Part model, mm, in its own coordinate system. Give positions to 0.01 mm unless a question says otherwise; leave off trailing zeros. Order: outer loops, then holes, each group sorted by start corner. A loop starts at its lowest first (then second) coordinate and runs counter-clockwise, first axis right, second up. Notation, with made-up numbers: M 76.5,-26 L 109.5,-26 A19 ccw 109.5,10 Z; hole C 17,-29.5 d10. An arc over 180 degrees is marked long. Answer as a JSON object with one key per item and string values.
Autodesk Inventor part; units mm, degrees
ref_plane "Work Plane2" through (191.5157, -160.0488, 0) normal (0.9992817, -0.0378944, 0) x (0.0378944, 0.9992817, 0)
ref_plane "YZ Plane" through (0, 0, 0) normal (1, 0, 0) x (0, 1, 0)
ref_plane "XZ Plane" through (0, 0, 0) normal (0, 1, 0) x (-1, 0, 0)
sketch "Sketch1" plane through (0, 0, 0) normal (0, 0, 1) x (1, 0, 0)
  circle A0 centre (0, 0) radius 6.05
surface extrude "ExtrusionSrf1" sketch "Sketch1" along normal mid plane 6 shown yes curves A0
sketch "Sketch2" plane through (0, 0, 0) normal (0, 0, 1) x (1, 0, 0)
  circle A0 centre (324.834, -10.3853) radius 6.05
  point P0 (0, 0)
surface extrude "ExtrusionSrf2" sketch "Sketch2" along normal mid plane 6 shown yes curves A0
sketch "Sketch3" plane through (0, 0, 0) normal (0, 0, 1) x (1, 0, 0)
  circle A0 centre (-9.3308, -291.8509) radius 6.11
  point P0 (0, 0)
surface extrude "ExtrusionSrf3" sketch "Sketch3" along normal blind 6 shown yes curves A0
sketch "Sketch4" plane through (0, 0, 0) normal (0, 0, 1) x (1, 0, 0)
  circle A0 centre (7.3217, -169.3662) radius 5.735
  point P0 (0, 0)
surface extrude "ExtrusionSrf4" sketch "Sketch4" along normal mid plane 6 shown yes curves A0
sketch "Sketch5" plane through (0, 0, 0) normal (0, 0, 1) x (1, 0, 0)
  circle A0 centre (319.839, -166.6212) radius 6.05
  point P0 (0, 0)
surface extrude "ExtrusionSrf5" sketch "Sketch5" along normal mid plane 6 shown yes curves A0
sketch "Sketch6" plane through (0, 0, 0) normal (0, 0, 1) x (1, 0, 0)
  circle A0 centre (160.3736, -162.9887) radius 3
  point P0 (0, 0)
surface extrude "ExtrusionSrf6" sketch "Sketch6" along normal mid plane 6 shown yes curves A0
sketch "Sketch7" plane through (0, 0, 0) normal (0, 0, 1) x (1, 0, 0)
  circle A0 centre (179.3639, -163.5958) radius 3
  point P0 (0, 0)
surface extrude "ExtrusionSrf7" sketch "Sketch7" along normal mid plane 6 shown yes curves A0
sketch "Sketch8" plane through (0, 0, 0) normal (0, 0, 1) x (1, 0, 0)
  circle A0 centre (0, 0) radius 6.05
  circle A1 centre (7.3217, -169.3662) radius 5.735
  circle A2 centre (-9.3308, -291.8509) radius 6.11
  circle A3 centre (160.3736, -162.9887) radius 3
  circle A4 centre (179.3639, -163.5958) radius 3
  circle A5 centre (319.839, -166.6212) radius 6.05
  circle A6 centre (324.834, -10.3853) radius 6.05
  arc A7 (0.2015, 6.3018) -> (-6.3017, 0.2028) centre (0, 0) ccw
  arc A8 (-15.6925, -291.6462) -> (-2.969, -292.0543) centre (-9.3308, -291.8509) ccw
  arc A9 (7.4878, -163.0034) -> (0.9599, -169.1628) centre (7.3217, -169.3662) ccw
  arc A10 (160.2691, -166.9923) -> (160.4782, -158.985) centre (160.3736, -162.9887) ccw
  arc A11 (331.1358, -10.5868) -> (325.0355, -4.0835) centre (324.834, -10.3853) ccw
  arc A12 (179.5157, -159.5937) -> (179.2122, -167.5979) centre (179.3639, -163.5958) ccw
  arc A13 (319.6001, -172.9217) -> (326.1408, -166.8227) centre (319.839, -166.6212) ccw
  line L0 (-15.6925, -291.6462) -> (-6.3017, 0.2028)
  line L1 (0.2015, 6.3018) -> (325.0355, -4.0835)
  line L2 (-2.969, -292.0543) -> (0.9599, -169.1628)
  line L3 (7.4878, -163.0034) -> (160.2691, -166.9923)
  line L4 (331.1358, -10.5868) -> (326.1408, -166.8227)
  line L5 (148.4782, -158.6717) -> (160.4782, -158.985)
  line L6 (179.2122, -167.5979) -> (319.6001, -172.9217)
  line L7 (179.5157, -159.5937) -> (191.5157, -160.0488)
  dimension "d14" = 0.255
  dimension "d15" = 0.255
  dimension "d16" = 0.255
  dimension "d17" = 0.63
  dimension "d19" = 0.255
  dimension "d22" = 1.005
  dimension "d23" = 1.005
  dimension "d35" = 12
  dimension "d36" = 12
ref_plane "Work Plane2" through (191.5157, -160.0488, 0) normal (0.9992817, -0.0378944, 0) x (0.0378944, 0.9992817, 0)
sketch "Sketch10" plane through (191.5157, -160.0488, 0) normal (0.9992817, -0.0378944, 0) x (0.0378944, 0.9992817, 0)
  line L0 (0.63, 3) -> (-0.255, 3)
  line L1 (-0.255, 3) -> (-0.255, -3)
  line L2 (-0.255, -3) -> (0.63, -3)
  line L3 (0.63, -3) -> (0.63, 3)
  line L4 (0.63, 0) -> (-0.255, 0) construction
  point P0 (152.6764, 0)
  point P1 (0, 0)
  dimension "d29" = 6
  dimension "d30" = 0.63
  dimension "d31" = 0.255
sweep "Sweep2" add profiles "Sketch10" path "Sketch8" path curves L7 A12 L6 A13 L4 A11 L1 A7 L0 A8 L2 A9 L3 A10 L5
equation "\"d14\" = inside"
equation "\"d15\" = inside"
equation "\"d16\" = inside"
equation "\"d17\" = backside"
equation "\"d19\" = inside"
equation "\"inside\" = 0.255"
equation "\"backside\" = 0.63"
properties part number "Belt 2" material "Rubber"
1. Cut at B-B on x = 196. Give the cut face in (y, z), plus the area to 3 significant figures.
Worked answers:
{"outline": "M -168.86,-3 L -167.98,-3 L -167.98,3 L -168.86,3 Z; M -0.21,-3 L 0.67,-3 L 0.67,3 L -0.21,3 Z", "area": "10.6 mm^2"}
2. Cut at C-C on y = -85. Give the cut face in (x, z).
Worked answers:
{"outline": "M -9.67,-3 L -8.79,-3 L -8.79,3 L -9.67,3 Z; M 328.5,-3 L 329.39,-3 L 329.39,3 L 328.5,3 Z"}
3. Probe line 1 along Y through (x, z) = (181.5, 1.05); line 2 along Y through (x, z) = (176, 2); line 3 along Y through (x, z) = (65, 2.05) (3 decimals). List the from-to ranges inside material, lowest first.
Worked answers:
{"line 1": "y = -168.32 to -167.43, -159.92 to -159.04, 0.25 to 1.14", "line 2": "y = -166.78 to -165.25, -161.94 to -160.41, 0.43 to 1.31", "line 3": "y = -165.135 to -164.25, 3.975 to 4.86"}
4. Pin check, flat tips, straight feed: P1, Ø1.5, axis at x = 235.5, z = 2, coming from the -Y side; P2, Ø2, axis at y = -196, z = 1.5, coming from the +X side; P3, Ø1.5, axis at y = -55.5, z = 0.5, coming from the +X side. Stop position of each tip, or through.
Worked answers:
{"P1": "stops at y = -170.39", "P2": "stops at x = 0.76", "P3": "stops at x = 330.35"}
